Design review of the part built by this model. Coordinates are the model's own, in mm. Round coordinates to 2 decimals unless told otherwise and drop trailing zeros. Order: outer loops, then holes, each group sorted by start corner. A loop starts at its lowest first (then second) coordinate and runs counter-clockwise, first axis right, second up. Notation, with made-up numbers: M 19.5,-10 L 27.5,-10 A30 cw 27.5,12 Z; hole C 25,49.5 d9. An arc over 180 degrees is marked long. Write item = value, one per line. Start each with the question number.
```python
from build123d import *

# Parameters (mm, degrees)
BOSS_EXTRUDE2_DEPTH = 1
SKETCH3_R           = 6
SKETCH3_R_2         = 2.15
CUT_EXTRUDE1_DEPTH  = 1
FILLET1_R           = 2
FILLET4_R           = 5


with BuildPart() as part:
    # Sketch1 → Boss-Extrude2 (new body)
    with BuildSketch(Plane(origin=(0, 0, 0), x_dir=(1, 0, 0), z_dir=(0, 1, 0))):
        with BuildLine():
            Line((-10.579737185, 4.699562588), (5.304686116, 9.105985786))
            add(Edge.make_bspline(
                [(5.304686116, 9.105985786), (17.993455135, 6.637762386), (10.246572083, -2.487952551)],
                knots=[0, 0, 0, 1, 1, 1], degree=2))
            Line((10.246572083, -2.487952551), (1.011646395, -8.037716806))
            Line((1.011646395, -8.037716806), (-10.959675931, -3.958567779))
            add(Edge.make_bspline(
                [(-10.579737185, 4.699562588), (-16.765680179, 0.278506662), (-10.959675931, -3.958567779)],
                knots=[0, 0, 0, 1, 1, 1], degree=2))
        make_face()
    extrude(amount=BOSS_EXTRUDE2_DEPTH)

    # Sketch3 → Cut-Extrude1 (cut)
    with BuildSketch(Plane(origin=(0, 1, 0), x_dir=(1, 0, 0), z_dir=(0, 1, 0))):
        with Locations(Location((0, 0, 0), (0, 0, 270))):
            Circle(SKETCH3_R)
        with Locations(Location((-10, 0, 0), (0, 0, 270))):
            Circle(SKETCH3_R_2)
        with Locations(Location((9.351513774, 3.542483611, 0), (0, 0, 270))):
            Circle(SKETCH3_R_2)
    extrude(amount=-CUT_EXTRUDE1_DEPTH, mode=Mode.SUBTRACT)

    # Fillet1
    fillet1_edges = [part.edges().sort_by_distance(p)[0] for p in [
        (1.011646395, 0.5, 8.037716806),
    ]]
    fillet(fillet1_edges, radius=FILLET1_R)

    # Fillet4
    fillet4_edges = [part.edges().sort_by_distance(p)[0] for p in [
        (5.304686116, 0.5, -9.105985786),
    ]]
    fillet(fillet4_edges, radius=FILLET4_R)


solid = part.part
```
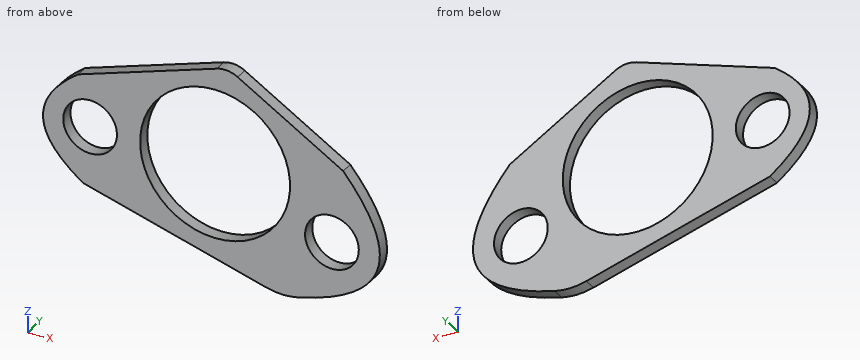
(1) For line 1 along X through (y, z) = (0.3, 0); line 2 along X through (y, z) = (0.5, 0.25); line 3 along X through (y, z) = (0.7, 2.25), list the stretches that pass through material, from the lowest coordinate up. Write a range as [from, to].
(2) Consider section A-A, the plane z = 5.5. Write out the cut boundary in (x, y).
(3) Consider section C-C, the plane z = -2.5. State how many separate pieces and enclosed holes the cut face has, then the cut area to 3 significant figures.
(4) Consider section B-B, the plane x = 2.75. Write out the cut boundary in (y, z), then the cut area to 3 significant figures.
(5) Insertion check: pin 1 (7 mm diameter, centred on x = 9.35, z = -3.54, fed in from +Y). The pin has a flat end and moves straight along its axis. Give the tip position at first contact, or say it passes through.
Completed:
q1.line_1 = [-13.77, -12.15], [-7.85, -6], [6, 12.05]
q1.line_2 = [-13.74, -12.14], [-7.86, -5.99], [5.99, 11.9]
q1.line_3 = [-12.81, -5.56], [5.56, 10.45]
q2.outline = M -6.44,0 L -2.4,0 L -2.4,1 L -6.44,1 Z; M 2.4,0 L 5.23,0 L 5.23,1 L 2.4,1 Z
q3.separate_pieces = 3
q3.enclosed_holes = 0
q3.area = 11.3 mm2
q4.outline = M 0,-8.4 L 1,-8.4 L 1,-5.33 L 0,-5.33 Z; M 0,5.33 L 1,5.33 L 1,6.99 L 0,6.99 Z
q4.area = 4.72 mm2
q5.pin_1 = 1
